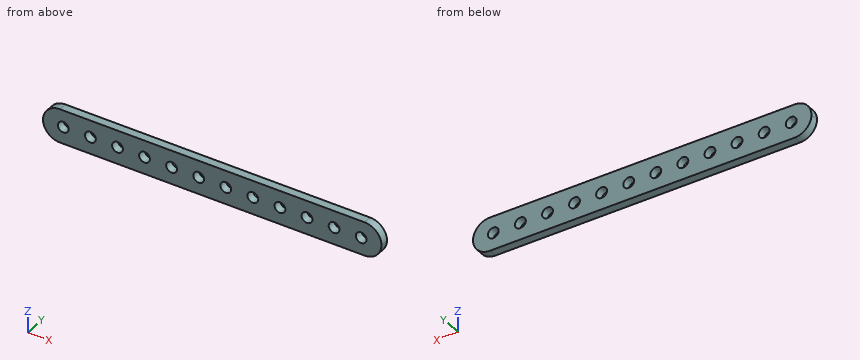
Autodesk Inventor part; units mm, degrees
ref_plane "YZ Plane" through (0, 0, 0) normal (1, 0, 0) x (0, 1, 0)
ref_plane "XZ Plane" through (0, 0, 0) normal (0, 1, 0) x (-1, 0, 0)
ref_plane "XY Plane" through (0, 0, 0) normal (0, 0, 1) x (1, 0, 0)
sketch "Sketch1" plane through (0, 0, 0) normal (0, 1, 0) x (-1, 0, 0)
  line L0 (-50, 0) -> (50, 0)
  line L1 (50, 0) -> (50, 10)
  line L2 (50, 10) -> (-50, 10)
  line L3 (-50, 10) -> (-50, 0)
  point P0 (0, 0)
  dimension "d0" = 10
  dimension "d1" = 100
  dimension "d2" = 50
extrude "Extrusion1" add sketch "Sketch1" along normal blind 2.5
sketch "Sketch2" plane through (0, 2.5, 0) normal (0, 1, 0) x (1, 0, 0)
  circle A0 centre (44, -5) radius 1.6
  line L0 (50, -10) -> (50, 0)
  line L1 (-50, -10) -> (50, -10)
  line L2 (50, 0) -> (-50, 0)
  line L3 (-50, 0) -> (-50, -10)
  circle A1 centre (36, -5) radius 1.6
  circle A2 centre (28, -5) radius 1.6
  circle A3 centre (20, -5) radius 1.6
  circle A4 centre (12, -5) radius 1.6
  circle A5 centre (4, -5) radius 1.6
  circle A6 centre (-4, -5) radius 1.6
  circle A7 centre (-12, -5) radius 1.6
  circle A8 centre (-20, -5) radius 1.6
  circle A9 centre (-28, -5) radius 1.6
  circle A10 centre (-36, -5) radius 1.6
  circle A11 centre (-44, -5) radius 1.6
  point P0 (0, 0)
  dimension "d5" = 6
  dimension "d6" = 3.2
  dimension "d7" = 10
  dimension "d8" = 5
  dimension "d10" = 100
  dimension "d13" = 8
  dimension "d18" = 6
extrude "Extrusion2" cut sketch "Sketch2" against normal through all contours A0 | A1 | A2 | A3 | A4 | A5 | A6 | A7 | A8 | A9 | A10 | A11
fillet "Fillet1" radius 5 4 edges at (50, 1.25, 10) (50, 1.25, 0) (-50, 1.25, 10) (-50, 1.25, 0)
equation "\"d8\" = 0.5 * d7"
properties part number "anchor-point"
Can you work these out from the model? Positions are in its coordinate system, mm. Give positions to 0.01 mm unless a question says otherwise; leave off trailing zeros. Write each loop counter-clockwise with the first axis right and the second up, starting at its lowest first coordinate (ties: lowest second). Pieces come first, ordered by that corner, then holes. Notation, with made-up numbers: (52.5, 0) -> (84.5, 0) arc R29 cw to (84.5, 22) -> close; hole circle Ø1 at (-16, -6.75). An arc over 180 degrees is marked (long way). Answer as a JSON object with one key per item and string values. Group by question number.
Item 1: Suppose I cut it at A-A (x = 36). Please give me the cut outline in (y, z).
Item 2: Suppose I cut it at B-B (y = 0.85). State how many separate pieces and enclosed holes the cut face has, plus the area to 3 significant figures.
Item 3: I'm going to push a flat-ended pin straight in: P1, Ø5, axis at x = -44, z = 5, coming from the -Y side. Where does the tip first touch, or does it pass through?
Item 4: Please list where these lines run through material, in increasing order: line 1 (Z direction, x = 36, y = 1.4); line 2 (Z direction, x = -44.5, y = 2.1); line 3 (X direction, y = 1.35, z = 1.25). Write a range as [from, to].
Findings:
{
 "1": {"outline": "(0, 0) -> (2.5, 0) -> (2.5, 3.4) -> (0, 3.4) -> close; (0, 6.6) -> (2.5, 6.6) -> (2.5, 10) -> (0, 10) -> close"},
 "2": {"separate pieces": "1", "enclosed holes": "12", "area": "882 mm²"},
 "3": {"P1": "stops at y = 0"},
 "4": {"line 1": "z = [0, 3.4], [6.6, 10]", "line 2": "z = [0, 3.48], [6.52, 10]", "line 3": "x = [-48.31, 48.31]"}
}
